```python
from build123d import *

# Parameters (mm, degrees)
F0_R     = 20
F1_DEPTH = 15
F2_R     = 18
F3_DEPTH = 13
F4_R     = 3.5
F4_R_2   = 1.5
F5_DEPTH = 16
F7_DEPTH = 2


with BuildPart() as f1:
    # F0 (on Top) → F1 (new body)
    with BuildSketch(Plane.XY):
        Circle(F0_R)
    extrude(amount=F1_DEPTH)

    # F2 (on face) → F3 (cut)
    with BuildSketch(Plane.XY.offset(15)):
        Circle(F2_R)
    extrude(amount=-F3_DEPTH, mode=Mode.SUBTRACT)

    # F4 (on face) → F5 (join)
    with BuildSketch(Plane.XY.offset(2)):
        Circle(F4_R)
        Circle(F4_R_2, mode=Mode.SUBTRACT)
    extrude(amount=F5_DEPTH)

    # F6 (on face) → F7 (cut)
    with BuildSketch(Plane.XY.offset(2)):
        with BuildLine():
            Line((-2.9187702811, 5.0554584226), (-1.8657855341, 17.9030400866))
            ThreePointArc((-1.8657855341, 17.9030400866), (-9, 15.5884572681), (-14.5715947529, 10.5673377138))
            Line((-14.5715947529, 10.5673377138), (-2.9187702811, 5.0554584226))
        make_face()
        with BuildLine():
            ThreePointArc((14.5715947529, 10.5673377138), (9, 15.5884572681), (1.8657855341, 17.9030400866))
            Line((1.8657855341, 17.9030400866), (2.9187702811, 5.0554584226))
            Line((2.9187702811, 5.0554584226), (14.5715947529, 10.5673377138))
        make_face()
        with BuildLine():
            ThreePointArc((18, 0), (17.6050112918, 3.7501436529), (16.437380287, 7.3357023728))
            Line((16.437380287, 7.3357023728), (5.8375405623, 0))
            Line((5.8375405623, 0), (16.437380287, -7.3357023728))
            ThreePointArc((16.437380287, -7.3357023728), (17.6050112918, -3.7501436529), (18, 0))
        make_face()
        with BuildLine():
            ThreePointArc((1.8657855341, -17.9030400866), (9, -15.5884572681), (14.5715947529, -10.5673377138))
            Line((14.5715947529, -10.5673377138), (2.9187702811, -5.0554584226))
            Line((2.9187702811, -5.0554584226), (1.8657855341, -17.9030400866))
        make_face()
        with BuildLine():
            Line((-2.9187702811, -5.0554584226), (-14.5715947529, -10.5673377138))
            ThreePointArc((-14.5715947529, -10.5673377138), (-9, -15.5884572681), (-1.8657855341, -17.9030400866))
            Line((-1.8657855341, -17.9030400866), (-2.9187702811, -5.0554584226))
        make_face()
        with BuildLine():
            Line((-5.8375405623, 0), (-16.437380287, 7.3357023728))
            ThreePointArc((-16.437380287, 7.3357023728), (-18, 0), (-16.437380287, -7.3357023728))
            Line((-16.437380287, -7.3357023728), (-5.8375405623, 0))
        make_face()
    extrude(amount=-F7_DEPTH, mode=Mode.SUBTRACT)


solid = f1.part
```
Design review of the part built by this model. Coordinates are the model's own, in mm. A direction names the side the tool comes from. Coordinates: 2 decimals unless noted, no trailing zeros. Order: outer loops, then holes, each group sorted by start corner. A loop starts at its lowest first (then second) coordinate and runs counter-clockwise, first axis right, second up.
1) Take a section at D-D, the plane x = 0. Give the boundary of the cut face in (y, z).
2) Take a section at B-B, the plane y = -6.5. Give the boundary of the cut face in (x, z).
3) Mouldability with a two-part tool opening along Y and no side actions: class faces 4 (the cylindrical face through (-4.336, -19.524, 7.395)), 5 (the flat face through (0, -2, 18)), 6 (the flat face through (2.4, -11.4, 1)), 7 (the cylindrical face through (-1.5, 0.07, 9.89)) as +Y half, -Y half, draft (parallel to the pull), parting line (faces both ways), or undercut.
4) Take a section at A-A, the plane z = 7.5. Give the boundary of the cut face in (x, y), and give its area (3 significant figures).
5) Clearance check with flat-ended pins moving along their axes: pin 1 (1.5 mm diameter, centred on x = -14.5, z = 10.5, fed in from -Y); pin 2 (8 mm diameter, centred on x = 10.5, z = 2.5, fed in from -Y); pin 3 (6 mm diameter, centred on x = 11, z = 8.5, fed in from -Y). State where each tip first meets the part, or that it passes through.
6) Take a section at C-C, the plane y = -16.5. Give the boundary of the cut face in (x, z).
7) For faces 1 (the flat face through (-11.21, -3.72, 1.01)), 2 (the cylindrical face through (3.233, -1.341, 9.888)), 3 (the flat face through (0, 0, 0)), list the 3-axis set-ups (+Z, -Z, +X, -X, +Y, -Y) from which the entire face can be reached by the end or side of a thin tool; tool diameter is ignored.
8) Wall thickness on line 1 along Y through (x, z) = (0, 11.25); line 2 along X through (y, z) = (10, 1); line 3 along Z through (x, y) = (0.5, -12.5): over which ranges is each line inside the solid? List them lowest first.
Returned:
1. outline: (-20, 0) - (20, 0) - (20, 15) - (18, 15) - (18, 2) - (3.5, 2) - (3.5, 18) - (1.5, 18) - (1.5, 2) - (-1.5, 2) - (-1.5, 18) - (-3.5, 18) - (-3.5, 2) - (-18, 2) - (-18, 15) - (-20, 15) - close
2. outline: (-18.91, 0) - (-16.79, 0) - (-16.79, 15) - (-18.91, 15) - close; (-15.23, 0) - (-5.97, 0) - (-5.97, 2) - (-15.23, 2) - close; (-2.8, 0) - (2.8, 0) - (2.8, 2) - (-2.8, 2) - close; (5.97, 0) - (15.23, 0) - (15.23, 2) - (5.97, 2) - close; (16.79, 0) - (18.91, 0) - (18.91, 15) - (16.79, 15) - close
3. face 4: parting line
3. face 5: draft
3. face 6: undercut
3. face 7: undercut
4. outline: circle Ø40 at (0, 0); circle Ø7 at (0, 0); hole circle Ø36 at (0, 0); hole circle Ø3 at (0, 0)
4. area: 270 mm2
5. pin 1: stops at y = -14.52
5. pin 2: stops at y = -18.91
5. pin 3: stops at y = -18.33
6. outline: (-11.3, 0) - (-7.19, 0) - (-7.19, 15) - (-11.3, 15) - close; (-1.98, 0) - (1.98, 0) - (1.98, 2) - (-1.98, 2) - close; (7.19, 0) - (11.3, 0) - (11.3, 15) - (7.19, 15) - close
7. face 1: +Z, -Z
7. face 2: +Z
7. face 3: -Z, +X, -X, +Y, -Y
8. line 1: y = -20 to -18, -3.5 to -1.5, 1.5 to 3.5, 18 to 20
8. line 2: x = -17.32 to -13.37, -2.51 to 2.51, 13.37 to 17.32
8. line 3: z = 0 to 2
